Check sheet for the drawn part. Datum: minimum x, y, z corner. Units: mm. A direction names the side the tool comes from. Coordinates: 2 decimals unless noted, no trailing zeros. Write each loop counter-clockwise with the first axis right and the second up, starting at its lowest first coordinate (ties: lowest second). Pieces come first, ordered by that corner, then holes. Notation, with made-up numbers: (30, 46) -> (44, 46) arc R10 ccw to (44, 52) -> close; hole circle Ø2 at (4, -2.5). An arc over 180 degrees is marked (long way). Answer in a Markdown table with one row per item. Add a question column.
Q1. Thickness scan on line 1 (Y direction, x = 5, z = 3.9); line 2 (Z direction, x = 8.5, y = 5.75); line 3 (Y direction, x = 2.75, z = 4.25) (1 decimal). Record the ranges inside material, lowest first.
Q2. Release check for a two-part mould opening along Y. For the marked faces 1, 2 and 3 record: pulls with the +Y half, pulls with the -Y half, needs draft (parallel to the pull), parting line crosses it, or undercut.
Q3. Gauge pin test, flat ends, axial feed: P1, Ø5, axis at x = 8.5, z = 2, coming from the -Y side; P2, Ø1, axis at y = 6, z = 5, coming from the +X side (3 decimals); P3, Ø2, axis at y = 2.5, z = 5, coming from the -X side; P4, Ø3, axis at y = 4.5, z = 8, coming from the -X side. Record the tip position at first contact, or that the pin passes through.
Q4. Section check A-A, the plane z = 4.25. Record the boundary of the cut face in (x, y), and give its area (3 significant figures).
Q5. Section check C-C, the plane z = 13.25. Record the boundary of the cut face in (x, y), and give its area (3 significant figures).
Q6. Section check B-B, the plane y = 9. Record the boundary of the cut face in (x, z), and give its area (3 significant figures).
Q7. Tool access check on the marked faces 4 and 5. Record the directions out of +Z, -Z, +X, -X, +Y, -Y that give a thin tool (end or side, any length) a straight path to the whole face; none if there is none.
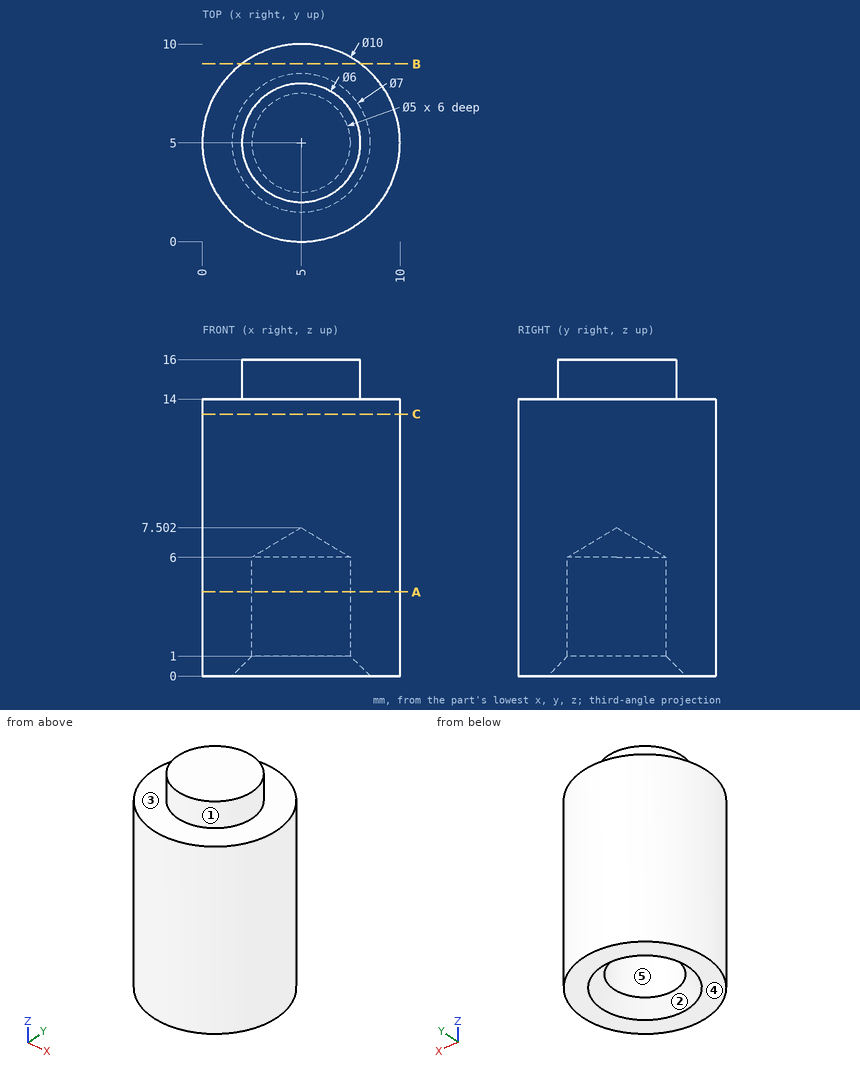
Calculated:
| question | item | result |
|---|---|---|
| 1 | line 1 | y = 0 to 2.5, 7.5 to 10 |
| 1 | line 2 | z = 0 to 14 |
| 1 | line 3 | y = 0.5 to 3.9, 6.1 to 9.5 |
| 2 | face 1 | parting line crosses it |
| 2 | face 2 | undercut |
| 2 | face 3 | needs draft |
| 3 | P1 | stops at y = 0.1 |
| 3 | P2 | stops at x = 9.975 |
| 3 | P3 | stops at x = 0.23 |
| 3 | P4 | stops at x = 0 |
| 4 | outline | circle Ø10 at (5, 5); hole circle Ø5 at (5, 5) |
| 4 | area | 58.9 mm² |
| 5 | outline | circle Ø10 at (5, 5) |
| 5 | area | 78.5 mm² |
| 6 | outline | (2, 0) -> (8, 0) -> (8, 14) -> (2, 14) -> close |
| 6 | area | 84.0 mm² |
| 7 | face 4 | -Z, +X, -X, +Y, -Y |
| 7 | face 5 | -Z |
